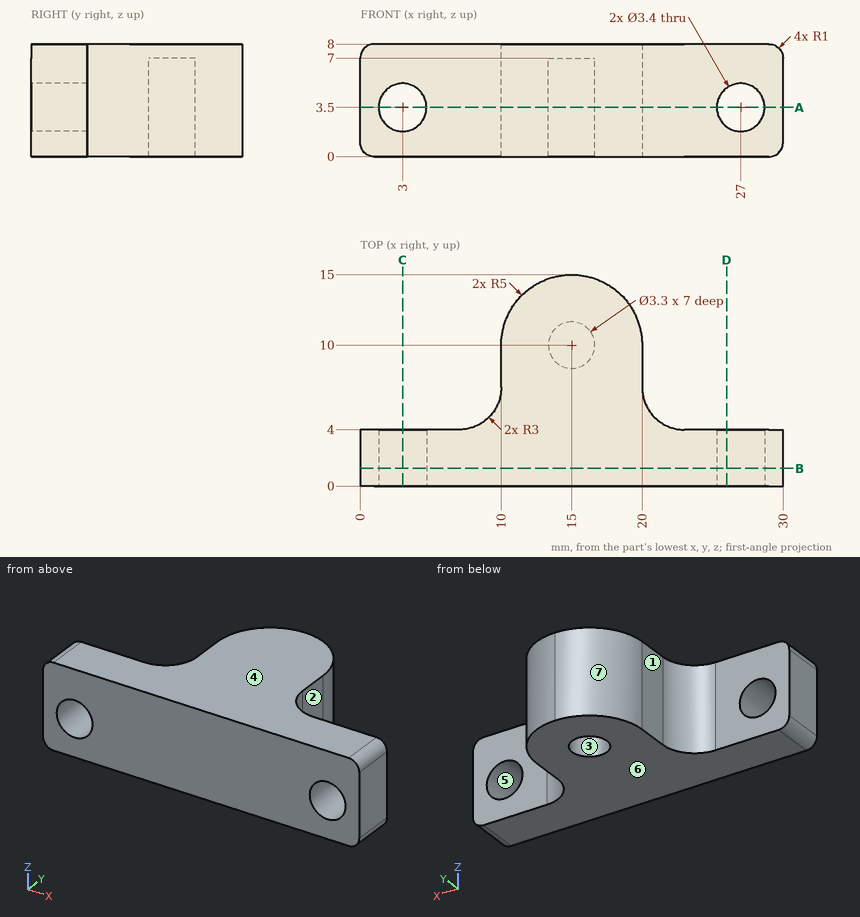
The drawing under review shows one solid part. Ordinate dimensions are in mm from its lowest x, y, z. A direction names the side the tool comes from. Round coordinates to 2 decimals unless told otherwise and drop trailing zeros. Loops run counter-clockwise (first coordinate to the right, second up) from the corner with the lowest first, then second, coordinate; pieces in that order, holes last. Notation, with made-up numbers: (30.25, 36) - (57.25, 36) arc R10 cw to (57.25, 51) - close; hole circle Ø8 at (49.25, -22.5). An arc over 180 degrees is marked (long way). One line per question, with ' | ' between items.
1. For the marked faces 1, 2 and 3, list the 3-axis set-ups (+Z, -Z, +X, -X, +Y, -Y) from which the entire face can be reached by the end or side of a thin tool; tool diameter is ignored.
Results are:
face 1: +Z, -Z, -X, +Y | face 2: +Z, -Z, +X, +Y | face 3: -Z
2. We need section A-A, the plane z = 3.5. State how many separate pieces and enclosed holes the cut face has, and give its area (3 significant figures).
Results are:
separate pieces: 3 | enclosed holes: 1 | area: 187 mm²
3. We need section C-C, the plane x = 3. State the section outline as (y, z) points.
Results are:
outline: (0, 0) - (4, 0) - (4, 1.8) - (0, 1.8) - close; (0, 5.2) - (4, 5.2) - (4, 8) - (0, 8) - close
4. We need section B-B, the plane y = 1.25. State the section outline as (x, z) points, and give its area (3 significant figures).
Results are:
outline: (0, 1) arc R1 ccw to (1, 0) - (29, 0) arc R1 ccw to (30, 1) - (30, 7) arc R1 ccw to (29, 8) - (1, 8) arc R1 ccw to (0, 7) - close; hole circle Ø3.4 at (3, 3.5); hole circle Ø3.4 at (27, 3.5) | area: 221 mm²
5. Clearance check with flat-ended pins moving along their axes: P1, Ø1.5, axis at y = 8.5, z = 2, coming from the +X side; P2, Ø2.5, axis at x = 27, z = 3.5, coming from the -Y side; P3, Ø0.9, axis at y = 9, z = 2, coming from the -X side; P4, Ø1, axis at y = 5.5, z = 4.5, coming from the +X side (1 decimal). State where each tip first meets the part, or that it passes through.
Results are:
P1: stops at x = 20 | P2: passes through | P3: stops at x = 10 | P4: stops at x = 20.8
6. For L1, parallel to Z at x = 27, y = 2.9; L2, parallel to X at y = 10, z = 1.75; L3, parallel to Y at x = 28.25, z = 1.25, list the stretches that pass through material, from the lowest coordinate up. Write a range as [from, to].
Results are:
L1: z = [0, 1.8], [5.2, 8] | L2: x = [10, 13.35], [16.65, 20] | L3: y = [0, 4]
7. Draft analysis for pull direction Z (two halves, no side actions). For the marked faces 4, 5, 6 and 7, state which applies: released by +Z, released by -Z, zero draft, split by the parting line, or undercut.
Results are:
face 4: released by +Z | face 5: undercut | face 6: released by -Z | face 7: zero draft
8. We need section D-D, the plane x = 26. State the section outline as (y, z) points (1 decimal).
Results are:
outline: (0, 0) - (4, 0) - (4, 2.1) - (0, 2.1) - close; (0, 4.9) - (4, 4.9) - (4, 8) - (0, 8) - close
